```python
from build123d import *

# Parameters (mm, degrees)
F1_DEPTH    = 3.175
F2_SIZE2    = 1.27
F2_SIZE     = 1.27
F3_SIZE     = 1.27
F4_T1_DEPTH = 11.3354455178
F5_R        = 1.27


# Not quite as in the source:
# - a fillet or chamfer that OpenCascade refuses, or shapes differently, is made with other operations: its cross-section is extruded or revolved along the edge and cut away or added


with BuildPart() as f1:
    # F0 (on Front) → F1 (new body, symmetric)
    with BuildSketch(Plane.XZ):
        with BuildLine():
            Line((-222.2856830398, -18.875252817), (58.6383169602, -18.875252817))
            Line((58.6383169602, -18.875252817), (60.004461396, -13.3959467614))
            ThreePointArc((60.004461396, -13.3959467614), (63.3823526363, -8.1944503889), (69.2465281888, -6.175252817))
            Line((69.2465281888, -6.175252817), (-217.0251707977, -6.175252817))
            Line((-217.0251707977, -6.175252817), (-222.2856830398, -18.875252817))
        make_face()
        Polygon((-255.1717254639, 14.010789607), (-222.2856830398, -18.875252817), (-217.0251707977, -6.175252817), (-238.4935903897, 15.293166775), align=None)
        with BuildLine():
            ThreePointArc((-22.1892522704, 31.924747183), (-139.0243312187, 27.4396580434), (-255.1717254639, 14.0107896071))
            Line((-255.1717254639, 14.0107896071), (-238.4935903897, 15.293166775))
            Line((-238.4935903897, 15.293166775), (-22.1892522704, 31.924747183))
        make_face()
        with BuildLine():
            Line((-238.4935903897, 15.293166775), (-217.0251707977, -6.175252817))
            Line((-217.0251707977, -6.175252817), (69.2465281888, -6.175252817))
            ThreePointArc((69.2465281888, -6.175252817), (76.7523306169, -9.8360772646), (78.4885949816, -18.0045588726))
            Line((78.4885949816, -18.0045588726), (76.6882737813, -25.225252817))
            Line((76.6882737813, -25.225252817), (86.5048686008, -25.225252817))
            Line((86.5048686008, -25.225252817), (88.3051898011, -18.0045588726))
            ThreePointArc((88.3051898011, -18.0045588726), (93.8510411727, -10.3362236111), (103.1599182919, -8.631923198))
            Line((103.1599182919, -8.631923198), (177.815158105, -23.8207034021))
            ThreePointArc((177.815158105, -23.8207034021), (183.9152537909, -27.983372217), (185.2067697838, -35.2546145785))
            Line((185.2067697838, -35.2546145785), (190.1425618478, -36.2588128234))
            Line((190.1425618478, -36.2588128234), (192.5143319625, -33.7604418083))
            Line((192.5143319625, -33.7604418083), (199.6791825839, -8.8887735704))
            Line((199.6791825839, -8.8887735704), (199.0935677301, -5.1867834867))
            Line((199.0935677301, -5.1867834867), (110.401744257, 21.506425589))
            ThreePointArc((110.401744257, 21.506425589), (103.0219894482, 27.389702526), (101.7390811386, 36.7399899454))
            Line((101.7390811386, 36.7399899454), (102.9133555046, 41.449747183))
            Line((102.9133555046, 41.449747183), (93.096760685, 41.449747183))
            Line((93.096760685, 41.449747183), (91.9221255914, 36.7385431459))
            ThreePointArc((91.9221255914, 36.7385431459), (89.6701980979, 33.2708788976), (85.7607477296, 31.924747183))
            Line((85.7607477296, 31.924747183), (-22.1892522704, 31.924747183))
            Line((-22.1892522704, 31.924747183), (-238.4935903897, 15.293166775))
        make_face()
        Polygon((202.0282745361, -23.738661781), (199.6791825839, -8.8887735704), (192.5143319625, -33.7604418083), align=None)
    extrude(amount=F1_DEPTH, both=True)

    # F2
    f2_edges = [f1.edges().sort_by_distance(p)[0] for p in [
        (93.096761, 0, 41.449747),
        (86.504869, 0, -25.225253),
    ]]
    chamfer(f2_edges, length=F2_SIZE, length2=F2_SIZE2)

    # F3
    f3_edges = [f1.edges().sort_by_distance(p)[0] for p in [
        (102.913356, 0, 41.449747),
        (76.688274, 0, -25.225253),
    ]]
    chamfer(f3_edges, length=F3_SIZE)

    # F4: chamfer of 1.016 on 1 edges, made by hand

    # F4_s2 → F4_t1 (cut)
    with BuildSketch(Plane.XZ.offset(-5.6677227589)):
        with BuildLine():
            Line((185.3423672188, -34.3154020779), (186.1779563064, -35.4804096602))
            Line((186.1779563064, -35.4804096602), (186.1739051499, -35.5003217302))
            ThreePointArc((186.1739051499, -35.5003217302), (185.6910670267, -35.3738822533), (185.2027186274, -35.2745266485))
            Line((185.2027186274, -35.2745266485), (185.1869498558, -35.2501343047))
            ThreePointArc((185.1869498558, -35.2501343047), (185.2797978886, -34.7859194498), (185.322207486, -34.3128550063))
            Line((185.322207486, -34.3128550063), (185.3423672188, -34.3154020779))
        make_face()
    extrude(amount=F4_T1_DEPTH, mode=Mode.SUBTRACT)

    # F5
    f5_edges = [f1.edges().sort_by_distance(p)[0] for p in [
        (202.028275, 0, -23.738662),
        (199.093568, 0, -5.186783),
        (190.142562, 0, -36.258813),
    ]]
    fillet(f5_edges, radius=F5_R)


solid = f1.part
```
Part model, mm, in its own coordinate system. Coordinates: 2 decimals unless noted, no trailing zeros. Write each loop counter-clockwise with the first axis right and the second up, starting at its lowest first coordinate (ties: lowest second). Pieces come first, ordered by that corner, then holes.
Item 1: Probe line 1 (Z direction, x = 12, y = 2.5); line 2 (Z direction, x = 98.5, y = -2.25). List the from-to ranges inside material, lowest first.
Item 2: Pin check, flat tip, straight feed: pin 1 (1.9 mm diameter, centred on x = -147.5, y = -0.5, fed in from -Z). Stop position of the tip, or through.
Item 3: Slice it at C-C (z = 1). Write the cut outline in (x, y) (3 decimals), and give its area (3 significant figures).
Item 4: Mould opens along X. For faces 1 (the face through (71.3, 0, -6.4)), 2 (the face through (103.09, -0.04, 27.27)), 3 (the face through (139.96, -0.04, -16.12)), 4 (the face through (-30, -3.175, 3)) say: released by +X, released by -X, zero draft, split by the parting line, or undercut.
Item 5: Slice it at B-B (x = 173). Write the cut outline in (y, z) (3 decimals), and give its area (3 significant figures).
Results found:
1. line 1: z = -18.88 to 31.92
1. line 2: z = -8.56 to 41.45
2. pin 1: stops at z = -18.88
3. outline: (-242.161, -3.175) - (178.537, -3.175) - (178.537, 3.175) - (-242.161, 3.175) - close
3. area: 2,670 mm2
4. face 1: undercut
4. face 2: released by +X
4. face 3: undercut
4. face 4: zero draft
5. outline: (-3.175, -22.841) - (3.175, -22.841) - (3.175, 2.666) - (-3.175, 2.666) - close
5. area: 162 mm2
